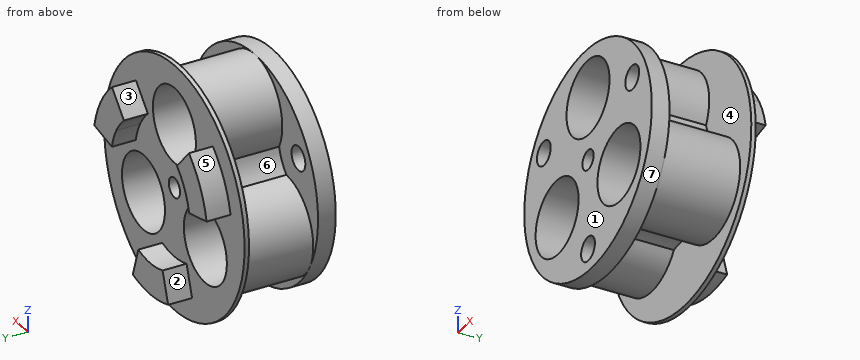
```python
from build123d import *

# Parameters (mm, degrees)
SKETCH1_R              = 27.5
SKETCH1_R_2            = 2.2
SKETCH1_R_3            = 8.425
BOSS_EXTRUDE1_DEPTH    = 22
BOSS_EXTRUDE2_DEPTH    = 5.4
CUT_EXTRUDE1_OUTLINE_R = 27.5
CUT_EXTRUDE1_DEPTH     = 17
SKETCH6_R              = 2.7
CUT_EXTRUDE2_DEPTH     = 5
SKETCH7_R              = 33.756466266
SKETCH7_R_2            = 27.5
SKETCH7_R_3            = 25
CUT_EXTRUDE6_DEPTH     = 4


# Read off the part's stored shape, not the designer's step: Cut-Extrude1
with BuildPart() as part:
    # Sketch1 → Boss-Extrude1 (new body)
    with BuildSketch(Plane(origin=(0, 0, 0), x_dir=(1, 0, 0), z_dir=(0, 1, 0))):
        with Locations(Location((0, 0, 0), (0, 0, 270))):
            Circle(SKETCH1_R)
        with Locations(Location((0, 0, 0), (0, 0, 270))):
            Circle(SKETCH1_R_2, mode=Mode.SUBTRACT)
        with Locations(Location((0, -14, 0), (0, 0, 270))):
            Circle(SKETCH1_R_3, mode=Mode.SUBTRACT)
        with Locations(Location((-12.124355653, 7, 0), (0, 0, 270))):
            Circle(SKETCH1_R_3, mode=Mode.SUBTRACT)
        with Locations(Location((12.124355653, 7, 0), (0, 0, 270))):
            Circle(SKETCH1_R_3, mode=Mode.SUBTRACT)
    extrude(amount=BOSS_EXTRUDE1_DEPTH)

    # Sketch4 → Boss-Extrude2 (add)
    with BuildSketch(Plane(origin=(0, 22, 0), x_dir=(1, 0, 0), z_dir=(0, 1, 0))):
        with BuildLine():
            ThreePointArc((-22.000122827, -4.716417665), (-19.485571585, -11.25), (-15.084598927, -16.694456422))
            Line((-15.084598927, -16.694456422), (-10.391612594, -11.500625535))
            ThreePointArc((-10.391612594, -11.500625535), (-13.423393759, -7.75), (-15.15564017, -3.249087725))
            Line((-15.15564017, -3.249087725), (-22.000122827, -4.716417665))
        make_face()
        with BuildLine():
            Line((4.764027576, 14.74971326), (6.9155239, 21.410874087))
            ThreePointArc((6.9155239, 21.410874087), (0, 22.5), (-6.9155239, 21.410874087))
            Line((-6.9155239, 21.410874087), (-4.764027576, 14.74971326))
            ThreePointArc((-4.764027576, 14.74971326), (0, 15.5), (4.764027576, 14.74971326))
        make_face()
        with BuildLine():
            Line((19.485571585, -11.25), (13.423393759, -7.75))
            ThreePointArc((13.423393759, -7.75), (12.054270192, -9.743950438), (10.391612594, -11.500625535))
            Line((10.391612594, -11.500625535), (15.084598927, -16.694456422))
            ThreePointArc((15.084598927, -16.694456422), (17.49813415, -14.144444184), (19.485571585, -11.25))
        make_face()
        with BuildLine():
            ThreePointArc((15.15564017, -3.249087725), (14.465643708, -5.567328992), (13.423393759, -7.75))
            Line((13.423393759, -7.75), (19.485571585, -11.25))
            ThreePointArc((19.485571585, -11.25), (20.998515061, -8.081606601), (22.000122827, -4.716417665))
            Line((22.000122827, -4.716417665), (15.15564017, -3.249087725))
        make_face()
    extrude(amount=BOSS_EXTRUDE2_DEPTH)

    # Cut-Extrude1 outline → Cut-Extrude1 (cut)
    with BuildSketch(Plane(origin=(0, 4, 0), x_dir=(1, 0, 0), z_dir=(0, 1, 0))):
        Circle(CUT_EXTRUDE1_OUTLINE_R)
        with BuildLine():
            ThreePointArc((12.609360996, -3.989302517), (10.825317547, -6.25), (9.759517821, -8.925375689))
            ThreePointArc((9.759517821, -8.925375689), (0, -25), (-9.759517821, -8.925375689))
            ThreePointArc((-9.759517821, -8.925375689), (-10.825317547, -6.25), (-12.609360996, -3.989302517))
            ThreePointArc((-12.609360996, -3.989302517), (-21.650635095, 12.5), (-2.849843175, 12.914678207))
            ThreePointArc((-2.849843175, 12.914678207), (0, 12.5), (2.849843175, 12.914678207))
            ThreePointArc((2.849843175, 12.914678207), (21.650635095, 12.5), (12.609360996, -3.989302517))
        make_face(mode=Mode.SUBTRACT)
    extrude(amount=CUT_EXTRUDE1_DEPTH, mode=Mode.SUBTRACT)

    # Sketch6 → Cut-Extrude2 (cut)
    with BuildSketch(Plane.XZ):
        with Locations(Location((0, -20, 0), (0, 0, 270))):
            Circle(SKETCH6_R)
        with Locations(Location((-17.320508076, 10, 0), (0, 0, 270))):
            Circle(SKETCH6_R)
        with Locations(Location((17.320508076, 10, 0), (0, 0, 270))):
            Circle(SKETCH6_R)
    extrude(amount=-CUT_EXTRUDE2_DEPTH, mode=Mode.SUBTRACT)

    # Sketch7 → Cut-Extrude6 (cut)
    # profile 1 of 2: a face of its own
    with BuildSketch(Plane.XZ):
        Circle(SKETCH7_R)
        with Locations(Location((0, 0, 0), (0, 0, 90))):
            Circle(SKETCH7_R_2, mode=Mode.SUBTRACT)
    # profile 2 of 2: a face of its own
    with BuildSketch(Plane.XZ):
        with Locations(Location((0, 0, 0), (0, 0, 90))):
            Circle(SKETCH7_R_2)
        with Locations(Location((0, 0, 0), (0, 0, 270))):
            Circle(SKETCH7_R_3, mode=Mode.SUBTRACT)
    extrude(amount=-CUT_EXTRUDE6_DEPTH, mode=Mode.SUBTRACT)


solid = part.part
```
CAD build for the part. Positions are in the model's coordinates, mm. Face numbers are marked on the shaded views. A direction names the side the tool comes from. Coordinates: 2 decimals unless noted, no trailing zeros. Order: outer loops, then holes, each group sorted by start corner. A loop starts at its lowest first (then second) coordinate and runs counter-clockwise, first axis right, second up. Notation, with made-up numbers: M 69,-12 L 103,-12 A13 ccw 103,2 Z; hole C -14,-20.5 d6. An arc over 180 degrees is marked long. Write each question's results on one line, items separated by ' | '. Start each with the question number.
Q1. Pull direction X, two halves, no side cores. Call the marked faces 1, 2 and 3: +X half, -X half, draft (parallel to the pull), parting line (faces both ways), or undercut.
Q2. Flat gauge pins, fed straight in: P1, Ø6, axis at y = 13.5, z = 2, coming from the -X side; P2, Ø3, axis at x = 0, z = -20, coming from the -Y side; P3, Ø1.5, axis at x = -16, y = 15.5, coming from the -Z side; P4, Ø6, axis at x = 17.32, z = 10, coming from the -Y side. Where does each tip first touch, or does it go through?
Q3. Cut at C-C (x = -1.5). List the corners of the cut face in (y, z) (3 decimals).
Q4. Drill centre lines: probe 1 along X at (y, z) = (16.5, -7.5); probe 2 along X at (y, z) = (7.5, -5); probe 3 along X at (y, z) = (1.15, 10). Where is each one in solid material? Low to high. Write a range as from..to.
Q5. Cut at A-A (y = 24.5). List the corners of the cut face in (x, z), then the cut area to 3 significant figures.
Q6. Which spindle directions (+Z, -Z, +X, -X, +Y, -Y) get a long thin tool onto all of the face, cutting with end or side? Do the marked faces 4, 5, 6 and 7. Say none if no direction does.
Found:
1) face 1: draft | face 2: -X half | face 3: undercut
2) P1: x = -21.34 | P2: y = 21 | P3: z = -17.55 | P4: y = 0
3) outline: M 0,-24.955 L 4,-24.955 L 4,-22.245 L 0,-22.245 Z; M 0,-17.755 L 4,-17.755 L 4,-12.613 L 21,-12.613 L 21,-27.459 L 22,-27.459 L 22,-22.45 L 27.4,-22.45 L 27.4,-15.427 L 22,-15.427 L 22,-1.609 L 0,-1.609 Z; M 0,1.609 L 22,1.609 L 22,5.71 L 0,5.71 Z; M 0,22.29 L 22,22.29 L 22,27.459 L 21,27.459 L 21,24.897 L 4,24.897 L 4,24.955 L 0,24.955 Z
4) probe 1: -23.11..-20.53, -3.71..3.71, 20.53..23.11 | probe 2: -22.94..-20.31, -3.94..3.94, 20.31..22.94 | probe 3: -22.91..-20.02, -14.62..-7.41, 7.41..14.62, 20.02..22.91
5) outline: M -22,4.72 L -15.16,3.25 A15.5 cw -10.39,11.5 L -15.08,16.69 A22.5 ccw Z; M -6.92,-21.41 A22.5 ccw 6.92,-21.41 L 4.76,-14.75 A15.5 cw -4.76,-14.75 Z; M 10.39,11.5 A15.5 cw 15.16,3.25 L 22,4.72 A22.5 ccw 15.08,16.69 Z | area: 249 mm²
6) face 4: none | face 5: +Z, -X, +Y | face 6: -X | face 7: -Y
